Can you work these out from the model? Positions are in its coordinate system, mm. A direction names the side the tool comes from. Give positions to 0.01 mm unless a question says otherwise; leave off trailing zeros. Loops run counter-clockwise (first coordinate to the right, second up) from the corner with the lowest first, then second, coordinate; pieces in that order, holes last.
from build123d import *

# Parameters (mm, degrees)
SKETCH1_R           = 23.5
BOSS_EXTRUDE1_DEPTH = 21.8
SKETCH2_W           = 20.417368514
SKETCH2_H           = 15.313025903
BOSS_EXTRUDE2_DEPTH = 2


with BuildPart() as part:
    # Sketch1 → Boss-Extrude1 (new body, symmetric)
    with BuildSketch(Plane(origin=(-36.272491561, 0, 0), x_dir=(-1, 0, 0), z_dir=(0, 0, -1))):
        with Locations((-36.272491561, 0)):
            Circle(SKETCH1_R)
    extrude(amount=BOSS_EXTRUDE1_DEPTH, both=True)

    # Sketch2 → Boss-Extrude2 (add)
    with BuildSketch(Plane.XY.offset(21.8)):
        with Locations((7.381083838, -21.231446412)):
            Rectangle(SKETCH2_W, SKETCH2_H)
    extrude(amount=-BOSS_EXTRUDE2_DEPTH)


solid = part.part
(1) Please list where these lines run through material, in increasing order: probe 1 along Y at (x, z) = (0, 10); probe 2 along X at (y, z) = (1.5, 11); probe 3 along X at (y, z) = (2, 13).
Returned:
probe 1: y = -23.5 to 23.5
probe 2: x = -23.45 to 23.45
probe 3: x = -23.41 to 23.41
(2) Will these pins go through, and if not, where does the flat tip stop? P1, Ø10, axis at x = 17.5, z = -15.5, coming from the +Y side; P2, Ø1.5, axis at y = -8.5, z = -16, coming from the -X side; P3, Ø8, axis at x = 10.5, z = 13, coming from the -Y side.
Returned:
P1: stops at y = 19.9
P2: stops at x = -22.19
P3: stops at y = -22.58
(3) Suppose I cut it at B-B on z = 9.5. List the corners of the cut face in (x, y) for me.
Returned:
outline: circle Ø47 at (0, 0)
(4) Suppose I cut it at A-A on x = 0. List the corners of the cut face in (y, z) for me, plus the area to 3 significant figures.
Returned:
outline: (-28.89, 19.8) - (-23.5, 19.8) - (-23.5, -21.8) - (23.5, -21.8) - (23.5, 21.8) - (-28.89, 21.8) - close
area: 2,060 mm2
(5) Suppose I cut it at D-D on y = -12. List the corners of the cut face in (x, z) for me, plus the area to 3 significant figures.
Returned:
outline: (-20.21, -21.8) - (20.21, -21.8) - (20.21, 21.8) - (-20.21, 21.8) - close
area: 1,760 mm2
(6) Suppose I cut it at C-C on y = -17.5. List the corners of the cut face in (x, z) for me, plus the area to 3 significant figures.
Returned:
outline: (-15.68, -21.8) - (15.68, -21.8) - (15.68, 19.8) - (17.59, 19.8) - (17.59, 21.8) - (-15.68, 21.8) - close
area: 1,370 mm2
(7) Which directions (+Z, -Z, +X, -X, +Y, -Y) give clear straight access to the entire face, cutting with the end or side of a thin tool? Please do faces 1 (the flat face through (-2.828, -26, 21)), 2 (the flat face through (7, -28.888, 21)), 3 (the flat face through (17.59, -22, 21)).
Returned:
face 1: +Z, -Z, -X, -Y
face 2: +Z, -Z, +X, -X, -Y
face 3: +Z, -Z, +X, -Y
